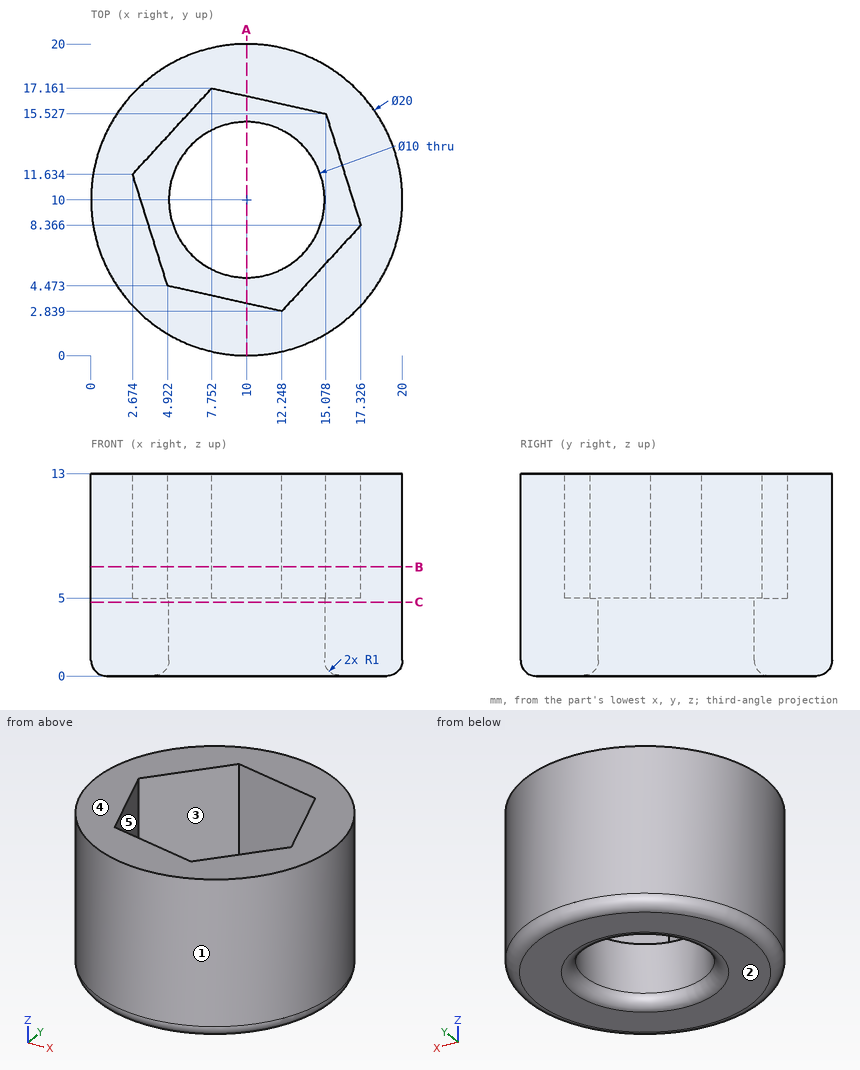
Design review of the part shown in the three views and the two pictorial views. Dimensions are in mm from the part's minimum x, y and z. A direction names the side the tool comes from. Give positions to 0.01 mm unless a question says otherwise; leave off trailing zeros. Write each loop counter-clockwise with the first axis right and the second up, starting at its lowest first coordinate (ties: lowest second). Pieces come first, ordered by that corner, then holes. Notation, with made-up numbers: (7, 8) - (65, 8) arc R27 ccw to (65, 35) - close; hole circle Ø8 at (5, 33.25). An arc over 180 degrees is marked (long way). Return JSON: item names as keys, results as strings. Group by question number.
(1) To check wall thickness, follow probe 1 along Y at (x, z) = (10, 3.3); probe 2 along X at (y, z) = (13.25, 10.5) (1 decimal); probe 3 along X at (y, z) = (18, 12.5). State the ranges of each line that lie inside material, in increasing order.
(2) Mouldability with a two-part tool opening along X and no side actions: class the marked faces 1, 2 and 3 as +X half, -X half, draft (parallel to the pull), parting line (faces both ways), or undercut.
(3) Machinability: for the marked faces 4 and 5, which of the approach directions +Z, -Z, +X, -X, +Y, -Y give a long, thin tool a straight path to every point of the face, cutting with its end or side? Answer none if there is none.
(4) Insertion check: pin 1 (3 mm diameter, centred on y = 17.5, z = 8, fed in from +X); pin 2 (5 mm diameter, centred on x = 6.5, z = 7.5, fed in from -Y). Each pin has a flat end and moves straight along its axis. Give the tip position at first contact, or say it passes through.
(5) We need section B-B, the plane z = 7. Give the boundary of the cut face in (x, y) (1 decimal), then the cut area to 3 significant figures.
(6) We need section C-C, the plane z = 4.75. Give the boundary of the cut face in (x, y), then the cut area to 3 significant figures.
(7) We need section A-A, the plane x = 10. Give the boundary of the cut face in (y, z), then the cut area to 3 significant figures.
Reported:
{
 "1": {"probe 1": "y = 0 to 5, 15 to 20", "probe 2": "x = 0.5 to 4.2, 15.8 to 19.5", "probe 3": "x = 4 to 16"},
 "2": {"face 1": "parting line", "face 2": "draft", "face 3": "undercut"},
 "3": {"face 4": "+Z, +X, -X, +Y, -Y", "face 5": "+Z"},
 "4": {"pin 1": "stops at x = 18", "pin 2": "stops at y = 0.05"},
 "5": {"outline": "circle Ø20 at (10, 10); hole (2.7, 11.6) - (4.9, 4.5) - (12.2, 2.8) - (17.3, 8.4) - (15.1, 15.5) - (7.8, 17.2) - close", "area": "168 mm2"},
 "6": {"outline": "circle Ø20 at (10, 10); hole circle Ø10 at (10, 10)", "area": "236 mm2"},
 "7": {"outline": "(0, 1) arc R1 ccw to (1, 0) - (4, 0) arc R1 ccw to (5, 1) - (5, 5) - (3.34, 5) - (3.34, 13) - (0, 13) - close; (15, 1) arc R1 ccw to (16, 0) - (19, 0) arc R1 ccw to (20, 1) - (20, 13) - (16.66, 13) - (16.66, 5) - (15, 5) - close", "area": "103 mm2"}
}
